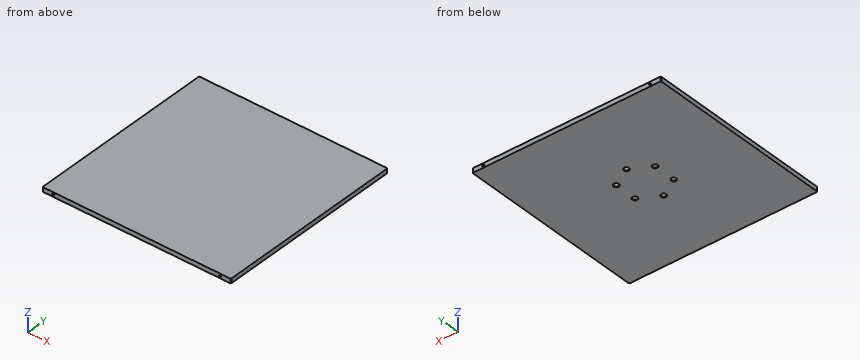
Autodesk Inventor part; units mm, degrees
ref_plane "Arbeitsebene2" through (-210, 0, 2.5) normal (-0.7054, 0.7088, 0) x (0.7088, 0.7054, 0)
ref_plane "Arbeitsebene3" through (-105, 0, 5) normal (1, 0, 0) x (0, 1, 0)
ref_plane "Arbeitsebene4" through (-210, 105, 5) normal (0, -1, 0) x (1, 0, 0)
sketch "Skizze3" plane through (0, 0, 0) normal (0, 0, 1) x (1, 0, 0)
  line L0 (0, 0) -> (-210, 0)
  line L1 (-210, 0) -> (-210, 210)
  line L2 (-210, 210) -> (0, 210)
  line L3 (0, 210) -> (0, 0)
  line L4 (0, 0) -> (-210, 210) construction
  line L5 (-210, 0) -> (0, 210) construction
  circle A0 centre (-105, 80) radius 2.5
  line L6 (-105, 58.1482) -> (-105, 151.8518) construction
  point P0 (-105, 105)
  point P1 (-105, 105)
  dimension "d4" = 210
  dimension "d5" = 210
  dimension "d10" = 5
  dimension "d11" = 25
extrude "Extrusion3" add sketch "Skizze3" along normal blind 5 contours L0 L1 L2 L3 | A0
fillet "Rundung1" radius 1 4 edges at (-210, 210, 2.5) (-210, 0, 2.5) (0, 0, 2.5) (0, 210, 2.5)
extrude "Extrusion4" cut sketch "Skizze3" along normal blind 4 contours A0
chamfer "Fase1" distance 0.5 angle 45 1 edges at (-107.5, 80, 0)
pattern_circular "Runde Anordnung1" count 6 over 360 about axis through (-105, 105, 0) along (0, 0, 1) of "Extrusion4", "Fase1"
sketch "Skizze5" plane through (-209, 0, 0) normal (0, -1, 0) x (1, 0, 0)
  line L0 (-1, 5) -> (-1, 0)
  line L1 (0, 0) -> (208, 0)
  line L2 (-2.4185, 2.5) -> (7.6142, 2.5) construction
  point P0 (209, 0)
  point P1 (11, 2.5)
  point P2 (-1, 2.5)
  dimension "d21" = 12
ref_plane "Arbeitsebene2" through (-210, 0, 2.5) normal (-0.7054, 0.7088, 0) x (0.7088, 0.7054, 0)
hole "Bohrung1" at (-198, 0, 2.5) direction (0, 1, 0) diameter 2.459 depth 8.8 tip angle 118
mirror "Spiegeln2" about plane through (-210, 0, 2.5) normal (-0.7054, 0.7088, 0) of "Bohrung1"
ref_plane "Arbeitsebene3" through (-105, 0, 5) normal (1, 0, 0) x (0, 1, 0)
ref_plane "Arbeitsebene4" through (-210, 105, 5) normal (0, -1, 0) x (1, 0, 0)
mirror "Spiegeln3" about plane through (-105, 0, 5) normal (1, 0, 0) of "Bohrung1", "Spiegeln2"
mirror "Spiegeln4" about plane through (-210, 105, 5) normal (0, -1, 0) of "Bohrung1", "Spiegeln2", "Spiegeln3"
equation "\"d5\" = d4"
properties part number "BT403_trajan20_21" material "Acryl"
Geometry: final body of the model. Coordinates: model frame, mm. Coordinates: 2 decimals unless noted, no trailing zeros. Order: outer loops, then holes, each group sorted by start corner. A loop starts at its lowest first (then second) coordinate and runs counter-clockwise, first axis right, second up.
1) First-contact query: P1, Ø2.5, axis at x = -83.5, y = 118.5, coming from the -Z side; P2, Ø4, axis at x = -104.5, y = 79.5, coming from the -Z side; P3, Ø2, axis at x = -198, z = 2.5, coming from the -Y side. Flat tips, straight axial feed; report the tip coordinate or a pass-through.
Result sheet:
P1: stops at z = 4
P2: stops at z = 0.29
P3: stops at y = 8.94
2) Section A-A (x = -105). Return loops of the section in (y, z), then the cut area to 3 significant figures.
Result sheet:
outline: (0, 0) - (77, 0) - (77.5, 0.5) - (77.5, 4) - (82.5, 4) - (82.5, 0.5) - (83, 0) - (127, 0) - (127.5, 0.5) - (127.5, 4) - (132.5, 4) - (132.5, 0.5) - (133, 0) - (210, 0) - (210, 5) - (0, 5) - close
area: 1,010 mm2
3) Section B-B (y = 130). Return loops of the section in (x, z).
Result sheet:
outline: (-210, 0) - (-108, 0) - (-107.5, 0.5) - (-107.5, 4) - (-102.5, 4) - (-102.5, 0.5) - (-102, 0) - (0, 0) - (0, 5) - (-210, 5) - close
4) Ray query, probe 1 along X at (y, z) = (207.25, 2.5); probe 2 along Z at (x, y) = (-198, 204); probe 3 along X at (y, z) = (81.5, 3.1). Return the intervals inside material, ascending.
Result sheet:
probe 1: x = -210 to -199.23, -196.77 to -13.23, -10.77 to 0
probe 2: z = 0 to 1.27, 3.73 to 5
probe 3: x = -210 to -107, -103 to 0
